Can you work these out from the model? Positions are in its coordinate system, mm. A direction names the side the tool comes from. Coordinates: 2 decimals unless noted, no trailing zeros.
```python
from build123d import *

# Parameters (mm, degrees)
SKETCH1_W               = 378
SKETCH1_H               = 16
BOSS_EXTRUDE1_DEPTH     = 6
CUT_EXTRUDE1_DEPTH      = 381.976768496
CUT_EXTRUDE1_DEPTH_BACK = 374
SKETCH3_W               = 4.3
SKETCH3_H               = 12.3
BOSS_EXTRUDE2_DEPTH     = 374
BOSS_EXTRUDE3_DEPTH     = 374
SKETCH6_W               = 4
SKETCH6_H               = 8.5
CUT_EXTRUDE2_DEPTH      = 378.00835287
SKETCH13_W              = 10
SKETCH13_H              = 15
BOSS_EXTRUDE5_DEPTH     = 4
FILLET10_R              = 4
SKETCH14_R              = 1.7
CUT_EXTRUDE5_DEPTH      = 4
FILLET11_R              = 4
FILLET12_R              = 4
LPATTERN3_COUNT         = 3
LPATTERN3_PITCH         = 172.5
LPATTERN4_COUNT         = 3
LPATTERN4_PITCH         = 172.5
FILLET13_R              = 4
FILLET14_R              = 4
FILLET16_R              = 4
FILLET17_R              = 4
FILLET18_R              = 4
FILLET19_R              = 4
FILLET20_R              = 2
FILLET21_R              = 2
FILLET22_R              = 2
SKETCH17_W              = 378
SKETCH17_H              = 16
BOSS_EXTRUDE6_DEPTH     = 6
FILLET25_R              = 4
SKETCH18_R              = 1
CUT_EXTRUDE6_DEPTH      = 0.7
FILLET26_R              = 0.5
FILLET27_R              = 0.5
SKETCH19_W              = 358
SKETCH19_H              = 6.3
CUT_EXTRUDE7_DEPTH      = 3
FILLET28_R              = 3


with BuildPart() as part:
    # Sketch1 → Boss-Extrude1 (new body)
    with BuildSketch(Plane.XY):
        with Locations((31.46991404, 39.151862464)):
            Rectangle(SKETCH1_W, SKETCH1_H)
    extrude(amount=BOSS_EXTRUDE1_DEPTH)

    # Sketch3 → Cut-Extrude1 (cut, two sides: drawn at the far end of the back side and taken through both)
    with BuildSketch(Plane(origin=(220.46991404, 0, 0), x_dir=(0, 0, -1), z_dir=(1, 0, 0)).offset(-CUT_EXTRUDE1_DEPTH_BACK)):
        with Locations((-3.85, 39.151862464)):
            Rectangle(SKETCH3_W, SKETCH3_H)
    extrude(amount=CUT_EXTRUDE1_DEPTH + CUT_EXTRUDE1_DEPTH_BACK, mode=Mode.SUBTRACT)

    # Sketch4 → Boss-Extrude2 (add)
    with BuildSketch(Plane(origin=(220.46991404, 0, 0), x_dir=(0, 0, -1), z_dir=(1, 0, 0))):
        Polygon((-6, 33.001862464), (-6, 34.001862464), (-5, 33.001862464), align=None)
    extrude(amount=-BOSS_EXTRUDE2_DEPTH)

    # Sketch5 → Boss-Extrude3 (add)
    with BuildSketch(Plane(origin=(220.46991404, 0, 0), x_dir=(0, 0, -1), z_dir=(1, 0, 0))):
        Polygon((-6, 45.301862464), (-6, 44.301862464), (-5, 45.301862464), align=None)
    extrude(amount=-BOSS_EXTRUDE3_DEPTH)

    # Sketch6 → Cut-Extrude2 (cut, through all)
    with BuildSketch(Plane(origin=(-153.53008596, 0, 0), x_dir=(0, 0, -1), z_dir=(1, 0, 0))):
        with Locations((-4, 39.151862464)):
            Rectangle(SKETCH6_W, SKETCH6_H)
    extrude(amount=-CUT_EXTRUDE2_DEPTH, mode=Mode.SUBTRACT)

    # Sketch13 → Boss-Extrude5 (add)
    with BuildSketch(Plane(origin=(0, 47.151862464, 0), x_dir=(1, 0, 0), z_dir=(0, 1, 0))):
        with Locations((-142.53008596, -7.5)):
            Rectangle(SKETCH13_W, SKETCH13_H)
    boss_extrude5 = extrude(amount=BOSS_EXTRUDE5_DEPTH)

    # Fillet10
    fillet10_edges = [part.edges().sort_by_distance(p)[0] for p in [
        (-142.53008596, 51.151862464, 0),
    ]]
    fillet(fillet10_edges, radius=FILLET10_R)

    # Sketch14 → Cut-Extrude5 (cut)
    with BuildSketch(Plane.XZ.offset(-47.151862464)):
        with Locations(Location((-142.53008596, 10, 0), (0, 0, 270))):
            Circle(SKETCH14_R)
    cut_extrude5 = extrude(amount=-CUT_EXTRUDE5_DEPTH, mode=Mode.SUBTRACT)

    # Fillet11
    fillet11_edges = [part.edges().sort_by_distance(p)[0] for p in [
        (-137.53008596, 49.151862464, 15),
    ]]
    fillet(fillet11_edges, radius=FILLET11_R)

    # Fillet12
    fillet12_edges = [part.edges().sort_by_distance(p)[0] for p in [
        (-147.53008596, 49.151862464, 15),
    ]]
    fillet(fillet12_edges, radius=FILLET12_R)

    # LPattern3: Boss-Extrude5 ×3
    with Locations(*[(i * LPATTERN3_PITCH, 0, 0) for i in range(1, LPATTERN3_COUNT)]):
        add(boss_extrude5)

    # LPattern4: Cut-Extrude5 ×3
    with Locations(*[(i * LPATTERN4_PITCH, 0, 0) for i in range(1, LPATTERN4_COUNT)]):
        add(cut_extrude5, mode=Mode.SUBTRACT)

    # Fillet13
    fillet13_edges = [part.edges().sort_by_distance(p)[0] for p in [
        (29.96991404, 51.151862464, 0),
    ]]
    fillet(fillet13_edges, radius=FILLET13_R)

    # Fillet14
    fillet14_edges = [part.edges().sort_by_distance(p)[0] for p in [
        (202.46991404, 51.151862464, 0),
    ]]
    fillet(fillet14_edges, radius=FILLET14_R)

    # Fillet16
    fillet16_edges = [part.edges().sort_by_distance(p)[0] for p in [
        (24.96991404, 49.151862464, 15),
    ]]
    fillet(fillet16_edges, radius=FILLET16_R)

    # Fillet17
    fillet17_edges = [part.edges().sort_by_distance(p)[0] for p in [
        (34.96991404, 49.151862464, 15),
    ]]
    fillet(fillet17_edges, radius=FILLET17_R)

    # Fillet18
    fillet18_edges = [part.edges().sort_by_distance(p)[0] for p in [
        (207.46991404, 49.151862464, 15),
    ]]
    fillet(fillet18_edges, radius=FILLET18_R)

    # Fillet19
    fillet19_edges = [part.edges().sort_by_distance(p)[0] for p in [
        (197.46991404, 49.151862464, 15),
    ]]
    fillet(fillet19_edges, radius=FILLET19_R)

    # Fillet20
    fillet20_edges = [part.edges().sort_by_distance(p)[0] for p in [
        (202.46991404, 47.151862464, 6),
    ]]
    fillet(fillet20_edges, radius=FILLET20_R)

    # Fillet21
    fillet21_edges = [part.edges().sort_by_distance(p)[0] for p in [
        (29.96991404, 47.151862464, 6),
    ]]
    fillet(fillet21_edges, radius=FILLET21_R)

    # Fillet22
    fillet22_edges = [part.edges().sort_by_distance(p)[0] for p in [
        (-142.53008596, 47.151862464, 6),
    ]]
    fillet(fillet22_edges, radius=FILLET22_R)

    # Sketch17 → Boss-Extrude6 (add)
    with BuildSketch(Plane(origin=(0, 0, 0), x_dir=(-1, 0, 0), z_dir=(0, 0, -1))):
        with Locations((-31.46991404, 39.151862464)):
            Rectangle(SKETCH17_W, SKETCH17_H)
    extrude(amount=BOSS_EXTRUDE6_DEPTH)

    # Fillet25
    fillet25_edges = [part.edges().sort_by_distance(p)[0] for p in [
        (220.46991404, 39.151862464, -6),
        (31.46991404, 31.151862464, -6),
        (-157.53008596, 39.151862464, -6),
        (31.46991404, 47.151862464, -6),
    ]]
    fillet(fillet25_edges, radius=FILLET25_R)

    # Sketch18 → Cut-Extrude6 (cut)
    with BuildSketch(Plane.XY.offset(1.7)):
        with Locations((218.46991404, 39.151862464)):
            Circle(SKETCH18_R)
    extrude(amount=-CUT_EXTRUDE6_DEPTH, mode=Mode.SUBTRACT)

    # Fillet26
    fillet26_edges = [part.edges().sort_by_distance(p)[0] for p in [
        (217.46991404, 39.151862464, 1.7),
    ]]
    fillet(fillet26_edges, radius=FILLET26_R)

    # Fillet27
    fillet27_edges = [part.edges().sort_by_distance(p)[0] for p in [
        (217.46991404, 39.151862464, 1),
    ]]
    fillet(fillet27_edges, radius=FILLET27_R)

    # Sketch19 → Cut-Extrude7 (cut)
    with BuildSketch(Plane.XY.offset(1.7)):
        with Locations((31.46991404, 39.151862464)):
            Rectangle(SKETCH19_W, SKETCH19_H)
    extrude(amount=-CUT_EXTRUDE7_DEPTH, mode=Mode.SUBTRACT)

    # Fillet28
    fillet28_edges = [part.edges().sort_by_distance(p)[0] for p in [
        (31.46991404, 42.301862464, -1.3),
        (210.46991404, 39.151862464, -1.3),
        (31.46991404, 36.001862464, -1.3),
        (-147.53008596, 39.151862464, -1.3),
    ]]
    fillet(fillet28_edges, radius=FILLET28_R - 0.0001)  # a hair under: the kernel refuses the full size


solid = part.part
```
1. I'm going to push flat-ended pins straight in: pin 1 (5 mm diameter, centred on x = 70.5, z = 6.5, fed in from +Y); pin 2 (3 mm diameter, centred on x = 90.5, y = 33, fed in from +Z); pin 3 (5 mm diameter, centred on x = -30.5, y = 47, fed in from -Z). Where does each tip first touch, or does it pass through?
Completed:
pin 1: stops at y = 47.15
pin 2: stops at z = 6
pin 3: stops at z = -5.77
2. Please list where these lines run through material, in increasing order: probe 1 along X at (y, z) = (49, 10); probe 2 along X at (y, z) = (47.75, 1); probe 3 along Y at (x, z) = (-22.5, 5).
Completed:
probe 1: x = -147.53 to -144.23, -140.83 to -137.53, 24.97 to 28.27, 31.67 to 34.97, 197.47 to 200.77, 204.17 to 207.47
probe 2: x = -147.53 to -137.53, 24.97 to 34.97, 197.47 to 207.47
probe 3: y = 31.15 to 33, 45.3 to 47.15
3. On a 3-axis mill with a long thin cutter (end or side, diameter ignored), from which of +Z, -Z, +X, -X, +Y, -Y can I reach the whole of each face in a straight line? I mean faces 1 (the flat face through (34, 39, -6)), 2 (the flat face through (30, 47.152, 12)). Say none if no direction works.
Completed:
face 1: -Z, +X, -X, +Y, -Y
face 2: +Z, +X, -X, -Y
4. Thinking about a two-plate mould opening in Y: for faces 3 (the flat face through (202, 47.152, 12)), 4 (the flat face through (207.47, 49, 6)), 5 (the flat face through (31, 43, 1.7)), which applies, pulls with the +Y half, pulls with the -Y half, needs draft (parallel to the pull), parting line crosses it, or undercut?
Completed:
face 3: pulls with the -Y half
face 4: needs draft
face 5: undercut
